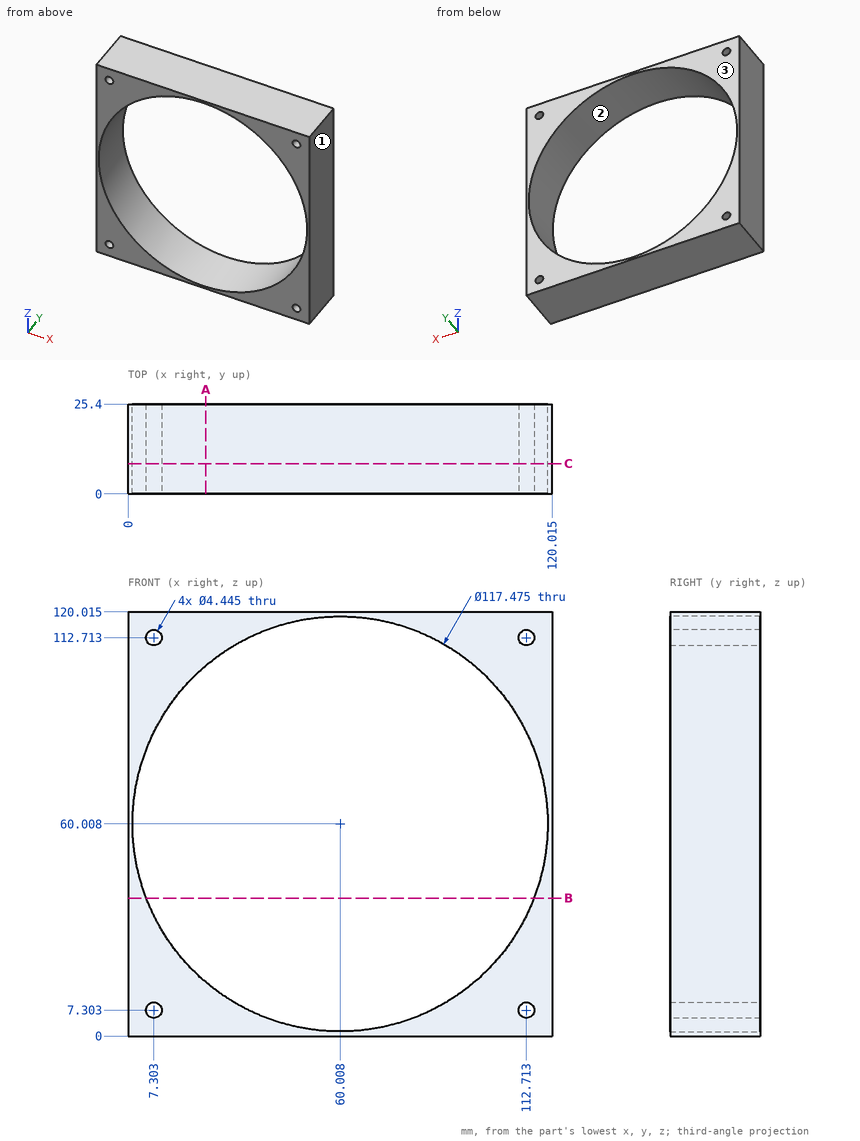
Input: dimensioned drawing with shaded views. Units: mm. Origin: part minimum x, y, z. Give positions to 0.01 mm unless a question says otherwise; leave off trailing zeros. Loops run counter-clockwise (first coordinate to the right, second up) from the corner with the lowest first, then second, coordinate; pieces in that order, holes last. Notation, with made-up numbers: (39, 39.25) - (57, 39.25) arc R13 ccw to (57, 52.25) - close; hole circle Ø9 at (9, -23). An arc over 180 degrees is marked (long way). Answer as CSV lines item,"result". Start each with the question number.
(1) Mould query, pull axis X, two halves, no side actions, for the marked faces 1, 2 and 3. Classes: +X half, -X half, draft (parallel to the pull), parting line (faces both ways), or undercut.
(2) Section query B-B (z = 39). Output: boundary loops of the cut face in (x, y) (1 decimal).
(3) Ray query, line 1 along X through (y, z) = (22.25, 59.5) (1 decimal); line 2 along Z through (x, y) = (14.5, 18) (1 decimal). Return the intervals inside material, ascending. Write a range as [from, to].
(4) Section query C-C (y = 8.5). Output: boundary loops of the cut face in (x, z) (1 decimal), and give its area (3 significant figures).
(5) Pin query (flat end, axial travel): P1, Ø5, axis at x = 7.3, z = 7.3, coming from the -Y side. Return the tip coordinate at first contact, or that it passes through.
(6) Section query A-A (x = 22). Output: boundary loops of the cut face in (y, z) (1 decimal).
Worked answers:
1,face 1,"+X half"
1,face 2,"undercut"
1,face 3,"draft"
2,outline,"(0, 0) - (5.2, 0) - (5.2, 25.4) - (0, 25.4) - close; (114.9, 0) - (120, 0) - (120, 25.4) - (114.9, 25.4) - close"
3,line 1,"x = [0, 1.3], [118.7, 120]"
3,line 2,"z = [0, 22.9], [97.1, 120]"
4,outline,"(0, 0) - (120, 0) - (120, 120) - (0, 120) - close; hole circle Ø117.5 at (60, 60); hole circle Ø4.4 at (7.3, 7.3); hole circle Ø4.4 at (7.3, 112.7); hole circle Ø4.4 at (112.7, 7.3); hole circle Ø4.4 at (112.7, 112.7)"
4,area,"3,500 mm^2"
5,P1,"stops at y = 0"
6,outline,"(0, 0) - (25.4, 0) - (25.4, 15.2) - (0, 15.2) - close; (0, 104.8) - (25.4, 104.8) - (25.4, 120) - (0, 120) - close"
